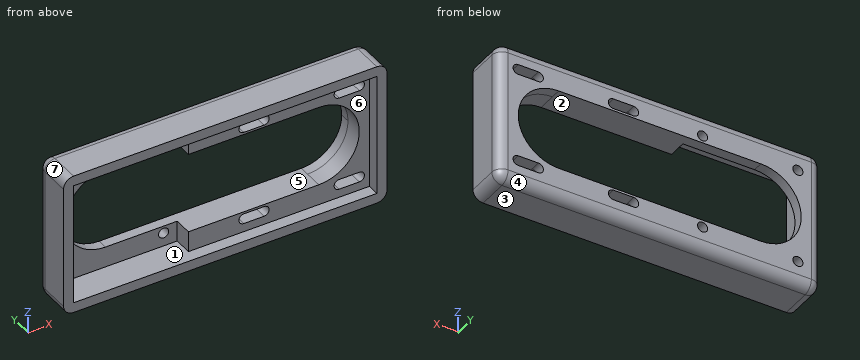
```python
from build123d import *

# Parameters (mm, degrees)
SKETCH2_R           = 2.5
SKETCH2_W           = 67
SKETCH2_H           = 1.75
BOSS_EXTRUDE1_DEPTH = 5
SKETCH4_W           = 160
SKETCH4_H           = 70.5
SKETCH4_W_2         = 150
SKETCH4_H_2         = 60.5
BOSS_EXTRUDE2_DEPTH = 20
SKETCH5_W           = 22.5
SKETCH5_H           = 10.25
BOSS_EXTRUDE3_DEPTH = 9
FILLET2_R           = 5


with BuildPart() as part:
    # Sketch2 → Boss-Extrude1 (new body)
    with BuildSketch(Plane(origin=(0, 0, 0), x_dir=(1, 0, 0), z_dir=(0, 1, 0))):
        with BuildLine():
            Line((-14.5, 30.25), (-75, 30.25))
            Line((-75, 30.25), (-75, -30.25))
            Line((-75, -30.25), (-14.5, -30.25))
            Line((-14.5, -30.25), (-14.5, -20))
            Line((-14.5, -20), (-50, -20))
            ThreePointArc((-50, -20), (-70, 0), (-50, 20))
            Line((-50, 20), (-14.5, 20))
            Line((-14.5, 20), (-14.5, 30.25))
        make_face()
        with Locations((-68.32, -23.57)):
            Circle(SKETCH2_R, mode=Mode.SUBTRACT)
        with Locations((-21.18, -23.57)):
            Circle(SKETCH2_R, mode=Mode.SUBTRACT)
        with Locations((-68.32, 23.57)):
            Circle(SKETCH2_R, mode=Mode.SUBTRACT)
        with Locations((-21.18, 23.57)):
            Circle(SKETCH2_R, mode=Mode.SUBTRACT)
        with BuildLine():
            Line((8, 30.25), (-14.5, 30.25))
            Line((-14.5, 30.25), (-14.5, 20))
            Line((-14.5, 20), (50, 20))
            ThreePointArc((50, 20), (64.142135624, 14.142135624), (70, 0))
            ThreePointArc((70, 0), (64.142135624, -14.142135624), (50, -20))
            Line((50, -20), (-14.5, -20))
            Line((-14.5, -20), (-14.5, -30.25))
            Line((-14.5, -30.25), (8, -30.25))
            Line((8, -30.25), (8, -28.5))
            Line((8, -28.5), (75, -28.5))
            Line((75, -28.5), (75, 28.5))
            Line((75, 28.5), (8, 28.5))
            Line((8, 28.5), (8, 30.25))
        make_face()
        with BuildLine():
            ThreePointArc((25.43, -23.57), (24.697766953, -25.337766953), (22.93, -26.07))
            Line((22.93, -26.07), (12.93, -26.07))
            ThreePointArc((12.93, -26.07), (10.43, -23.57), (12.93, -21.07))
            Line((12.93, -21.07), (22.93, -21.07))
            ThreePointArc((22.93, -21.07), (24.697766953, -21.802233047), (25.43, -23.57))
        make_face(mode=Mode.SUBTRACT)
        with BuildLine():
            ThreePointArc((72.57, -23.57), (71.837766953, -25.337766953), (70.07, -26.07))
            Line((70.07, -26.07), (60.07, -26.07))
            ThreePointArc((60.07, -26.07), (57.57, -23.57), (60.07, -21.07))
            Line((60.07, -21.07), (70.07, -21.07))
            ThreePointArc((70.07, -21.07), (71.837766953, -21.802233047), (72.57, -23.57))
        make_face(mode=Mode.SUBTRACT)
        with BuildLine():
            ThreePointArc((25.43, 23.57), (24.697766953, 21.802233047), (22.93, 21.07))
            Line((22.93, 21.07), (12.93, 21.07))
            ThreePointArc((12.93, 21.07), (10.43, 23.57), (12.93, 26.07))
            Line((12.93, 26.07), (22.93, 26.07))
            ThreePointArc((22.93, 26.07), (24.697766953, 25.337766953), (25.43, 23.57))
        make_face(mode=Mode.SUBTRACT)
        with BuildLine():
            ThreePointArc((60.07, 21.07), (57.57, 23.57), (60.07, 26.07))
            Line((60.07, 26.07), (70.07, 26.07))
            ThreePointArc((70.07, 26.07), (71.837766953, 25.337766953), (72.57, 23.57))
            ThreePointArc((72.57, 23.57), (71.837766953, 21.802233047), (70.07, 21.07))
            Line((70.07, 21.07), (60.07, 21.07))
        make_face(mode=Mode.SUBTRACT)
        with Locations((41.5, -29.375)):
            Rectangle(SKETCH2_W, SKETCH2_H)
        with Locations((41.5, 29.375)):
            Rectangle(SKETCH2_W, SKETCH2_H)
    extrude(amount=BOSS_EXTRUDE1_DEPTH)

    # Sketch4 → Boss-Extrude2 (add)
    with BuildSketch(Plane(origin=(0, 5, 0), x_dir=(1, 0, 0), z_dir=(0, 1, 0))):
        Rectangle(SKETCH4_W, SKETCH4_H)
        Rectangle(SKETCH4_W_2, SKETCH4_H_2, mode=Mode.SUBTRACT)
    extrude(amount=-BOSS_EXTRUDE2_DEPTH)

    # Sketch5 → Boss-Extrude3 (add)
    with BuildSketch(Plane(origin=(0, 0, 0), x_dir=(-1, 0, 0), z_dir=(0, -1, 0))):
        with BuildLine():
            Line((-8, 20), (-8, 30.25))
            Line((-8, 30.25), (-75, 30.25))
            Line((-75, 30.25), (-75, -30.25))
            Line((-75, -30.25), (-8, -30.25))
            Line((-8, -30.25), (-8, -20))
            Line((-8, -20), (-50, -20))
            ThreePointArc((-50, -20), (-70, 0), (-50, 20))
            Line((-50, 20), (-8, 20))
        make_face()
        with BuildLine():
            ThreePointArc((-57.57, -23.57), (-58.302233047, -25.337766953), (-60.07, -26.07))
            Line((-60.07, -26.07), (-70.07, -26.07))
            ThreePointArc((-70.07, -26.07), (-72.57, -23.57), (-70.07, -21.07))
            Line((-70.07, -21.07), (-60.07, -21.07))
            ThreePointArc((-60.07, -21.07), (-58.302233047, -21.802233047), (-57.57, -23.57))
        make_face(mode=Mode.SUBTRACT)
        with BuildLine():
            ThreePointArc((-10.43, -23.57), (-11.162233047, -25.337766953), (-12.93, -26.07))
            Line((-12.93, -26.07), (-22.93, -26.07))
            ThreePointArc((-22.93, -26.07), (-25.43, -23.57), (-22.93, -21.07))
            Line((-22.93, -21.07), (-12.93, -21.07))
            ThreePointArc((-12.93, -21.07), (-11.162233047, -21.802233047), (-10.43, -23.57))
        make_face(mode=Mode.SUBTRACT)
        with BuildLine():
            ThreePointArc((-70.07, 21.07), (-72.57, 23.57), (-70.07, 26.07))
            Line((-70.07, 26.07), (-60.07, 26.07))
            ThreePointArc((-60.07, 26.07), (-58.302233047, 25.337766953), (-57.57, 23.57))
            ThreePointArc((-57.57, 23.57), (-58.302233047, 21.802233047), (-60.07, 21.07))
            Line((-60.07, 21.07), (-70.07, 21.07))
        make_face(mode=Mode.SUBTRACT)
        with BuildLine():
            ThreePointArc((-22.93, 21.07), (-25.43, 23.57), (-22.93, 26.07))
            Line((-22.93, 26.07), (-12.93, 26.07))
            ThreePointArc((-12.93, 26.07), (-11.162233047, 25.337766953), (-10.43, 23.57))
            ThreePointArc((-10.43, 23.57), (-11.162233047, 21.802233047), (-12.93, 21.07))
            Line((-12.93, 21.07), (-22.93, 21.07))
        make_face(mode=Mode.SUBTRACT)
        with Locations((3.25, 25.125)):
            Rectangle(SKETCH5_W, SKETCH5_H)
        with Locations((3.25, -25.125)):
            Rectangle(SKETCH5_W, SKETCH5_H)
    extrude(amount=BOSS_EXTRUDE3_DEPTH)

    # Fillet2
    fillet2_edges = [part.edges().sort_by_distance(p)[0] for p in [
        (-80, 5, 0),
        (0, 5, 35.25),
        (0, 5, -35.25),
        (-80, -5, -35.25),
        (80, 5, 0),
        (80, -5, -35.25),
        (80, -5, 35.25),
        (-80, -5, 35.25),
    ]]
    fillet(fillet2_edges, radius=FILLET2_R)


solid = part.part
```
Source: CAD feature listing. Evaluate the final solid. Frame: model axes, mm. Face numbers are marked on the shaded views. A direction names the side the tool comes from. Coordinates: 2 decimals unless noted, no trailing zeros. Write each loop counter-clockwise with the first axis right and the second up, starting at its lowest first coordinate (ties: lowest second). Pieces come first, ordered by that corner, then holes. Notation, with made-up numbers: (49.5, -5) -> (53.5, -5) arc R30 ccw to (53.5, 28) -> close; hole circle Ø9 at (9, 36). An arc over 180 degrees is marked (long way). Return JSON: item names as keys, results as strings. Group by question number.
1) Section query D-D, the plane y = -5.25. State how many separate pieces and enclosed holes the cut face has, plus the area to 3 significant figures.
2) Section query C-C, the plane x = -22. Return loops of the section in (y, z), plus the area to 3 significant figures.
3) Set-up query: the marked faces 1, 2 and 3. Return all of +Z, -Z, +X, -X, +Y, -Y with unobstructed straight access to the full face (end or side cutting, diameter ignored); none if empty.
4) Ray query, line 1 along Z through (x, y) = (17, -4); line 2 along Z through (x, y) = (-19, -6.75); line 3 along X through (y, z) = (-10.75, 4). Return the intervals inside material, ascending.
5) Section query A-A, the plane z = 12. Return loops of the section in (x, y), plus the area to 3 significant figures.
6) Mould query, pull axis X, two halves, no side actions, for the marked faces 4, 5, 6 and 7. Classes: +X half, -X half, draft (parallel to the pull), parting line (faces both ways), or undercut.
7) Section query B-B, the plane x = -62. Return loops of the section in (y, z).
From the geometry:
{
 "1": {"separate pieces": "1", "enclosed holes": "5", "area": "4,110 mm²"},
 "2": {"outline": "(-15, -35.25) -> (0, -35.25) arc R5 ccw to (5, -30.25) -> (5, -25.93) -> (0, -25.93) -> (0, -30.25) -> (-15, -30.25) -> close; (-15, 30.25) -> (0, 30.25) -> (0, 25.93) -> (5, 25.93) -> (5, 30.25) arc R5 ccw to (0, 35.25) -> (-15, 35.25) -> close; (0, -21.21) -> (5, -21.21) -> (5, -20) -> (0, -20) -> close; (0, 20) -> (5, 20) -> (5, 21.21) -> (0, 21.21) -> close", "area": "245 mm²"},
 "3": {"face 1": "-Y", "face 2": "+Y, -Y", "face 3": "-Z, +X, -X, +Y, -Y"},
 "4": {"line 1": "-35.25 to -26.07, -21.07 to -20, 20 to 21.07, 26.07 to 35.25", "line 2": "-35.25 to -30.25, 30.25 to 35.25", "line 3": "-80 to -75, 75 to 80"},
 "5": {"outline": "(-80, -15) -> (-75, -15) -> (-75, 0) -> (-66, 0) -> (-66, 5) -> (-75, 5) arc R5 ccw to (-80, 0) -> close; (66, -9) -> (75, -9) -> (75, -15) -> (80, -15) -> (80, 0) arc R5 ccw to (75, 5) -> (66, 5) -> close", "area": "360 mm²"},
 "6": {"face 4": "draft", "face 5": "undercut", "face 6": "undercut", "face 7": "-X half"},
 "7": {"outline": "(-15, -35.25) -> (0, -35.25) arc R5 ccw to (5, -30.25) -> (5, -16) -> (0, -16) -> (0, -30.25) -> (-15, -30.25) -> close; (-15, 30.25) -> (0, 30.25) -> (0, 16) -> (5, 16) -> (5, 30.25) arc R5 ccw to (0, 35.25) -> (-15, 35.25) -> close"}
}
